CAD build for the part. Positions are in the model's coordinates, mm. A direction names the side the tool comes from. Round coordinates to 2 decimals unless told otherwise and drop trailing zeros. Loops run counter-clockwise (first coordinate to the right, second up) from the corner with the lowest first, then second, coordinate; pieces in that order, holes last.
```python
from build123d import *

# Parameters (mm, degrees)
F0_R     = 1.5
F0_R_2   = 4
F1_DEPTH = 3


with BuildPart() as f1:
    # F0 (on Top) → F1 (new body)
    with BuildSketch(Plane.XY):
        with BuildLine():
            Line((0, 90), (-39.499227, 90))
            ThreePointArc((-39.499227, 90), (-43.155307, 90.223615), (-46.756884, 90.891128))
            Line((-46.756884, 90.891128), (-85.364324, 100.517044))
            ThreePointArc((-85.364324, 100.517044), (-100.517044, 91.412371), (-91.412371, 76.259651))
            Line((-91.412371, 76.259651), (-65.161562, 69.714589))
            ThreePointArc((-65.161562, 69.714589), (-54.239785, 62.621904), (-50, 50.308675))
            Line((-50, 50.308675), (-50, 0))
            Line((-50, 0), (0, 0))
            Line((0, 0), (0, 73.5))
            ThreePointArc((0, 73.5), (-1.5, 75), (0, 76.5))
            Line((0, 76.5), (0, 90))
        make_face()
        with Locations((-35, 40)):
            Circle(F0_R, mode=Mode.SUBTRACT)
        with Locations((-96.531437, 83.495486)):
            Circle(F0_R, mode=Mode.SUBTRACT)
        with Locations((-84.268043, 81.531009)):
            Circle(F0_R, mode=Mode.SUBTRACT)
        with Locations((-88.388348, 88.388348)):
            Circle(F0_R_2, mode=Mode.SUBTRACT)
        with Locations((-92.508652, 95.245686)):
            Circle(F0_R, mode=Mode.SUBTRACT)
        with Locations((-80.245258, 93.281209)):
            Circle(F0_R, mode=Mode.SUBTRACT)
        with BuildLine():
            Line((39.499227, 90), (0, 90))
            Line((0, 90), (0, 76.5))
            ThreePointArc((0, 76.5), (1.06066, 76.06066), (1.5, 75))
            ThreePointArc((1.5, 75), (1.06066, 73.93934), (0, 73.5))
            Line((0, 73.5), (0, 0))
            Line((0, 0), (50, 0))
            Line((50, 0), (50, 50.308675))
            ThreePointArc((50, 50.308675), (54.239785, 62.621904), (65.161562, 69.714589))
            Line((65.161562, 69.714589), (91.412371, 76.259651))
            ThreePointArc((91.412371, 76.259651), (100.517044, 91.412371), (85.364324, 100.517044))
            Line((85.364324, 100.517044), (46.756884, 90.891128))
            ThreePointArc((46.756884, 90.891128), (43.155307, 90.223615), (39.499227, 90))
        make_face()
        with Locations((35, 40)):
            Circle(F0_R, mode=Mode.SUBTRACT)
        with Locations((84.268043, 81.531009)):
            Circle(F0_R, mode=Mode.SUBTRACT)
        with Locations((96.531437, 83.495486)):
            Circle(F0_R, mode=Mode.SUBTRACT)
        with Locations((80.245258, 93.281209)):
            Circle(F0_R, mode=Mode.SUBTRACT)
        with Locations((88.388348, 88.388348)):
            Circle(F0_R_2, mode=Mode.SUBTRACT)
        with Locations((92.508652, 95.245686)):
            Circle(F0_R, mode=Mode.SUBTRACT)
        with BuildLine():
            Line((0, -73.5), (0, 0))
            Line((0, 0), (-50, 0))
            Line((-50, 0), (-50, -50.308675))
            ThreePointArc((-50, -50.308675), (-54.239785, -62.621904), (-65.161562, -69.714589))
            Line((-65.161562, -69.714589), (-91.412371, -76.259651))
            ThreePointArc((-91.412371, -76.259651), (-100.517044, -91.412371), (-85.364324, -100.517044))
            Line((-85.364324, -100.517044), (-46.756884, -90.891128))
            ThreePointArc((-46.756884, -90.891128), (-43.155307, -90.223615), (-39.499227, -90))
            Line((-39.499227, -90), (0, -90))
            Line((0, -90), (0, -76.5))
            ThreePointArc((0, -76.5), (-1.5, -75), (0, -73.5))
        make_face()
        with Locations((-92.508652, -95.245686)):
            Circle(F0_R, mode=Mode.SUBTRACT)
        with Locations((-88.388348, -88.388348)):
            Circle(F0_R_2, mode=Mode.SUBTRACT)
        with Locations((-80.245258, -93.281209)):
            Circle(F0_R, mode=Mode.SUBTRACT)
        with Locations((-96.531437, -83.495486)):
            Circle(F0_R, mode=Mode.SUBTRACT)
        with Locations((-84.268043, -81.531009)):
            Circle(F0_R, mode=Mode.SUBTRACT)
        with BuildLine():
            Line((50, 0), (0, 0))
            Line((0, 0), (0, -73.5))
            ThreePointArc((0, -73.5), (1.06066, -73.93934), (1.5, -75))
            ThreePointArc((1.5, -75), (1.06066, -76.06066), (0, -76.5))
            Line((0, -76.5), (0, -90))
            Line((0, -90), (39.499227, -90))
            ThreePointArc((39.499227, -90), (43.155307, -90.223615), (46.756884, -90.891128))
            Line((46.756884, -90.891128), (85.364324, -100.517044))
            ThreePointArc((85.364324, -100.517044), (100.517044, -91.412371), (91.412371, -76.259651))
            Line((91.412371, -76.259651), (65.161562, -69.714589))
            ThreePointArc((65.161562, -69.714589), (54.239785, -62.621904), (50, -50.308675))
            Line((50, -50.308675), (50, 0))
        make_face()
        with Locations((80.245258, -93.281209)):
            Circle(F0_R, mode=Mode.SUBTRACT)
        with Locations((92.508652, -95.245686)):
            Circle(F0_R, mode=Mode.SUBTRACT)
        with Locations((88.388348, -88.388348)):
            Circle(F0_R_2, mode=Mode.SUBTRACT)
        with Locations((84.268043, -81.531009)):
            Circle(F0_R, mode=Mode.SUBTRACT)
        with Locations((96.531437, -83.495486)):
            Circle(F0_R, mode=Mode.SUBTRACT)
    extrude(amount=-F1_DEPTH)


solid = f1.part
```
Item 1: Cut at A-A, the plane x = -72.5. Give the cut face in (y, z), plus the area to 3 significant figures.
Answers follow:
outline: (-97.31, -3) - (-71.54, -3) - (-71.54, 0) - (-97.31, 0) - close; (71.54, -3) - (97.31, -3) - (97.31, 0) - (71.54, 0) - close
area: 155 mm2
Item 2: Cut at B-B, the plane y = -20.5. Give the cut face in (x, z).
Answers follow:
outline: (-50, -3) - (50, -3) - (50, 0) - (-50, 0) - close
Item 3: Flat gauge pins, fed straight in: P1, Ø6.5, axis at x = -88.39, y = 88.39, coming from the +Z side; P2, Ø0.9, axis at y = -1.5, z = -1.5, coming from the -X side; P3, Ø1, axis at y = -61, z = -1, coming from the +X side; P4, Ø0.9, axis at y = 5, z = -1.5, coming from the +X side. Where does each tip first touch, or does it go through?
Answers follow:
P1: passes through
P2: stops at x = -50
P3: stops at x = 53.42
P4: stops at x = 50
Item 4: Cut at D-D, the plane z = -1.4. State how many separate pieces and enclosed holes the cut face has, plus the area to 3 significant figures.
Answers follow:
separate pieces: 1
enclosed holes: 24
area: 22,800 mm2
Item 5: 3-axis set-ups, long thin cutter, end or side, ignore diameter. For faces 5 (the cylindrical face through (-54.13, -62.48, -1.48)), 6 (the flat face through (66.33, 95.77, -1.48)), 7 (the cylindrical face through (54.13, 62.48, -1.48)): which of +Z, -Z, +X, -X, +Y, -Y reach the whole face in a straight line?
Answers follow:
face 5: +Z, -Z, -X
face 6: +Z, -Z, +Y
face 7: +Z, -Z, +X
Item 6: Probe line 1 (Y direction, x = -86, z = -2.35); line 2 (Y direction, x = 87, z = -2.8); line 3 (X direction, y = -4.5, z = -1.9). List the from-to ranges inside material, lowest first.
Answers follow:
line 1: y = -100.66 to -91.6, -85.18 to -74.91, 74.91 to 85.18, 91.6 to 100.66
line 2: y = -100.81 to -92.14, -84.64 to -75.16, 75.16 to 84.64, 92.14 to 100.81
line 3: x = -50 to 50
Item 7: Two-plate mould, pull along X, no slides. Class faces 1 (the flat face through (78.471, -73.033, -1.479)), 2 (the flat face through (-1, 1, -3)), 3 (the flat face through (-78.471, 73.033, -1.479)), 4 (the cylindrical face through (-84.57, -87.19, -1.48)): released by +X, released by -X, zero draft, split by the parting line, or undercut.
Answers follow:
face 1: released by +X
face 2: zero draft
face 3: released by -X
face 4: undercut
Item 8: Cut at C-C, the plane x = -19.5. Give the cut face in (y, z), plus the area to 3 significant figures.
Answers follow:
outline: (-90, -3) - (90, -3) - (90, 0) - (-90, 0) - close
area: 540 mm2
